Verification items for this drawing (mm, ordinates from the low corner). A direction names the side the tool comes from. Round coordinates to 2 decimals unless told otherwise and drop trailing zeros. Write each loop counter-clockwise with the first axis right and the second up, starting at its lowest first coordinate (ties: lowest second). Pieces come first, ordered by that corner, then holes. Notation, with made-up numbers: (-0.5, 4.25) -> (27.5, 4.25) arc R36 ccw to (27.5, 38.25) -> close; hole circle Ø4 at (-40, 81.25). An arc over 180 degrees is marked (long way). One line per item, written item: value.
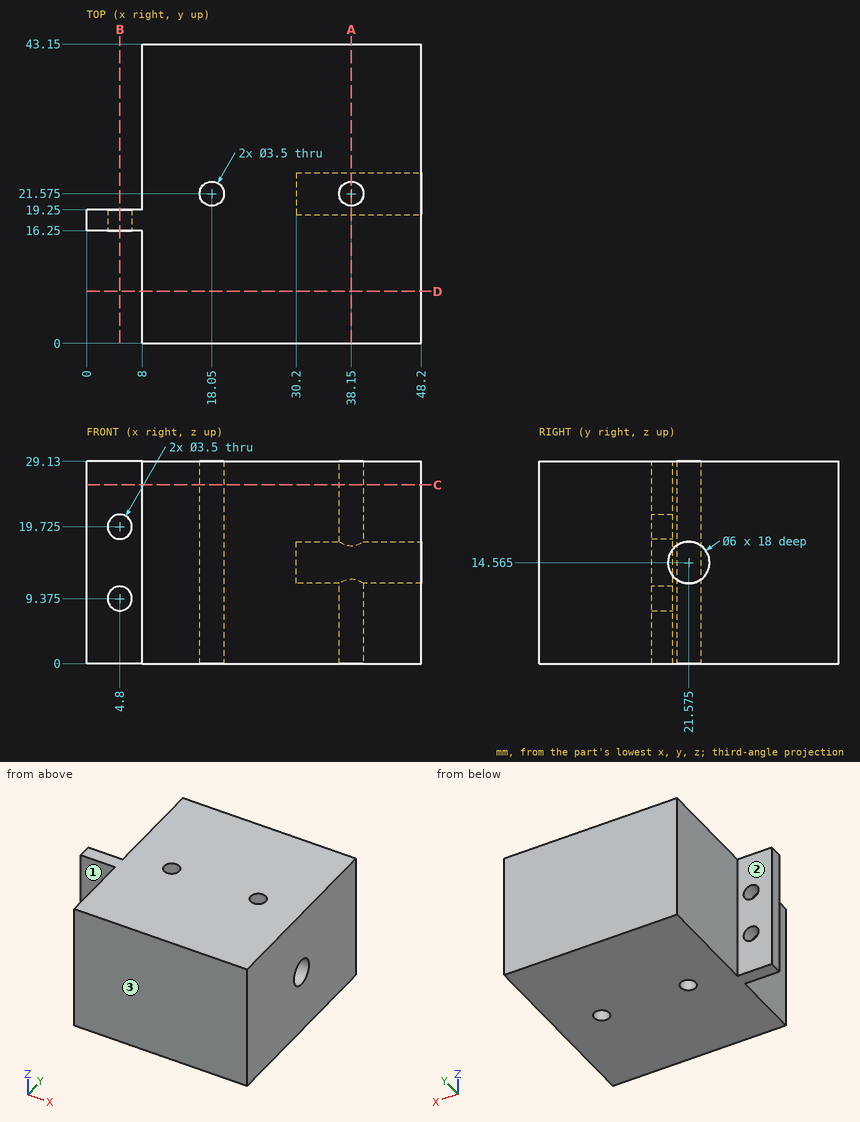
Item 1: Sectioned sample at D-D (y = 7.5). Enter the section's corners in (x, z).
Result set:
outline: (8, 0) -> (48.2, 0) -> (48.2, 29.13) -> (8, 29.13) -> close
Item 2: Sectioned sample at C-C (z = 25.75). Enter the section's corners in (x, y) (3 decimals).
Result set:
outline: (0, 16.25) -> (8, 16.25) -> (8, 0) -> (48.2, 0) -> (48.2, 43.15) -> (8, 43.15) -> (8, 19.25) -> (0, 19.25) -> close; hole circle Ø3.5 at (18.05, 21.575); hole circle Ø3.5 at (38.15, 21.575)
Item 3: Tool access check on the marked faces 1, 2 and 3. Record the directions out of +Z, -Z, +X, -X, +Y, -Y that give a thin tool (end or side, any length) a straight path to the whole face; none if there is none.
Result set:
face 1: +Z, -Z, -X, -Y
face 2: +Z, -Z, -X, +Y
face 3: +Z, -Z, +X, -X, -Y
Item 4: Sectioned sample at B-B (x = 4.8). Enter the section's corners in (y, z) (3 decimals).
Result set:
outline: (16.25, 0) -> (19.25, 0) -> (19.25, 7.625) -> (16.25, 7.625) -> close; (16.25, 11.125) -> (19.25, 11.125) -> (19.25, 17.975) -> (16.25, 17.975) -> close; (16.25, 21.475) -> (19.25, 21.475) -> (19.25, 29.13) -> (16.25, 29.13) -> close
Item 5: Depth check by flat-ended pin: pin 1 (1 mm diameter, centred on y = 27, z = 25, fed in from -X); pin 2 (6.5 mm diameter, centred on x = 2.5, z = 8, fed in from -Y); pin 3 (1.8 mm diameter, centred on y = 22.5, z = 15, fed in from +X). Enter the tip coordinate at first touch or a pass-through.
Result set:
pin 1: x = 8
pin 2: y = 16.25
pin 3: x = 30.2
Item 6: Sectioned sample at A-A (x = 38.15). Enter the section's corners in (y, z) (3 decimals), then the cut area to 3 significant figures.
Result set:
outline: (0, 0) -> (19.825, 0) -> (19.825, 12.128) arc R3 cw to (19.825, 17.002) -> (19.825, 29.13) -> (0, 29.13) -> close; (23.325, 0) -> (43.15, 0) -> (43.15, 29.13) -> (23.325, 29.13) -> (23.325, 17.002) arc R3 cw to (23.325, 12.128) -> close
area: 1,150 mm^2
Item 7: Material ranges on line 1 along Z through (x, y) = (4.8, 17) (3 decimals); line 2 along Z through (x, y) = (4, 18); line 3 along Y through (x, z) = (38, 19), recorded low to high.
Result set:
line 1: 0 to 7.625, 11.125 to 17.975, 21.475 to 29.13
line 2: 0 to 7.82, 10.93 to 18.17, 21.28 to 29.13
line 3: 0 to 19.83, 23.32 to 43.15
